Geometry check sheet. Reference: the model listing, model coordinates, mm. A direction names the side the tool comes from. Round coordinates to 2 decimals unless told otherwise and drop trailing zeros. Write each loop counter-clockwise with the first axis right and the second up, starting at its lowest first coordinate (ties: lowest second). Pieces come first, ordered by that corner, then holes. Notation, with made-up numbers: (66.25, -36) -> (100.25, -36) arc R15 ccw to (100.25, -19) -> close; hole circle Ø11 at (65, 75.25). An arc over 180 degrees is marked (long way). Use a Markdown table: item, result.
```python
from build123d import *

# Parameters (mm, degrees)
SKETCH1_R           = 12.5
BOSS_EXTRUDE1_DEPTH = 17.5
SKETCH2_R           = 2
BOSS_EXTRUDE2_DEPTH = 26
CHAMFER1_SIZE       = 10
SKETCH3_W           = 28.997372317
SKETCH3_H           = 7.197339184
CUT_EXTRUDE1_DEPTH  = 20
SKETCH4_R           = 5
CUT_EXTRUDE2_DEPTH  = 5
SKETCH5_R           = 3.5
BOSS_EXTRUDE3_DEPTH = 3.5
CUT_EXTRUDE6_START  = -1
CUT_EXTRUDE6_DEPTH  = 1


with BuildPart() as part:
    # Sketch1 → Boss-Extrude1 (new, symmetric)
    with BuildSketch(Plane(origin=(0, 0, 0), x_dir=(0, 0, -1), z_dir=(1, 0, 0))):
        Circle(SKETCH1_R)
    extrude(amount=BOSS_EXTRUDE1_DEPTH, both=True)

    # Sketch2 → Boss-Extrude2 (add, symmetric)
    with BuildSketch(Plane(origin=(0, 0, 0), x_dir=(0, 0, -1), z_dir=(1, 0, 0))):
        with Locations(Location((0, 0, 0), (0, 0, 180))):
            Circle(SKETCH2_R)
    extrude(amount=BOSS_EXTRUDE2_DEPTH, both=True)

    # Chamfer1
    chamfer1_edges = [part.edges().sort_by_distance(p)[0] for p in [
        (-17.5, 0, 12.5),
        (17.5, 0, 12.5),
    ]]
    chamfer(chamfer1_edges, length=CHAMFER1_SIZE)

    # Sketch3 → Cut-Extrude1 (cut, symmetric)
    with BuildSketch(Plane(origin=(0, 0, 0), x_dir=(0, 0, -1), z_dir=(1, 0, 0))):
        with Locations((0.644848308, -13.770631617)):
            Rectangle(SKETCH3_W, SKETCH3_H)
    extrude(amount=CUT_EXTRUDE1_DEPTH, both=True, mode=Mode.SUBTRACT)

    # Sketch4 → Cut-Extrude2 (cut)
    with BuildSketch(Plane.XZ.offset(10.171962025)):
        with Locations(Location((0, 0, 0), (0, 0, 270))):
            Circle(SKETCH4_R)
    extrude(amount=-CUT_EXTRUDE2_DEPTH, mode=Mode.SUBTRACT)

    # Sketch5 → Boss-Extrude3 (add)
    with BuildSketch(Plane.ZY.offset(26)):
        Circle(SKETCH5_R)
    boss_extrude3 = extrude(amount=BOSS_EXTRUDE3_DEPTH)

    # Sketch6 → Cut-Extrude6 (cut)
    with BuildSketch(Plane.ZY.offset(29.5).offset(CUT_EXTRUDE6_START)):
        with BuildLine():
            Line((2.803043133, -2.095936352), (-2.095936352, 2.803043133))
            ThreePointArc((-2.095936352, 2.803043133), (-2.474873734, 2.474873734), (-2.803043133, 2.095936352))
            Line((-2.803043133, 2.095936352), (2.095936352, -2.803043133))
            ThreePointArc((2.095936352, -2.803043133), (2.474873734, -2.474873734), (2.803043133, -2.095936352))
        make_face()
    cut_extrude6 = extrude(amount=CUT_EXTRUDE6_DEPTH, mode=Mode.SUBTRACT)

    # Mirror1: Boss-Extrude3, Cut-Extrude6 across plane
    add(boss_extrude3.mirror(Plane(origin=(0, 0, 0), x_dir=(0, 0, 1), z_dir=(1, 0, 0))))
    add(cut_extrude6.mirror(Plane(origin=(0, 0, 0), x_dir=(0, 0, 1), z_dir=(1, 0, 0))), mode=Mode.SUBTRACT)


solid = part.part
```
(1) Section check C-C on x = -22.5. Record the cut outline in (y, z), plus the area to 3 significant figures.
A:
| item | result |
|---|---|
| outline | circle Ø4 at (0, 0) |
| area | 12.6 mm2 |
(2) Thickness scan on line 1 (X direction, y = -8.3, z = 0); line 2 (X direction, y = -6.4, z = 0); line 3 (Y direction, x = 23, z = 1.25). Record the ranges inside material, lowest first.
A:
| item | result |
|---|---|
| line 1 | x = -11.7 to -5, 5 to 11.7 |
| line 2 | x = -13.6 to -5, 5 to 13.6 |
| line 3 | y = -1.56 to 1.56 |
(3) Release check for a two-part mould opening along Y. For faces 6 (the face through (28.993, 0.319, 0.388)), 7 (the face through (0, -5.172, 0)), 8 (the face through (-27.726, -3.105, 1.615)) record: +Y half, -Y half, draft (parallel to the pull), parting line (faces both ways), or undercut.
A:
| item | result |
|---|---|
| face 6 | undercut |
| face 7 | -Y half |
| face 8 | parting line |
(4) Gauge pin test, flat ends, axial feed: pin 1 Ø3 at (x, z) = (-8, 4.5) entering from +Y; pin 2 Ø12 at (x, z) = (17, -7) entering from +Y; pin 3 Ø6 at (x, y) = (-4.5, -2) entering from +Z; pin 4 Ø2 at (y, z) = (-7.5, -8) entering from -X. Record the tip position at first contact, or that the pin passes through.
A:
| item | result |
|---|---|
| pin 1 | stops at y = 12.11 |
| pin 2 | stops at y = 7.17 |
| pin 3 | stops at z = 12.5 |
| pin 4 | stops at x = -10.03 |
(5) Section check D-D on x = -11.5. Record the cut outline in (y, z), plus the area to 3 significant figures.
A:
| item | result |
|---|---|
| outline | circle Ø17 at (0, 0) |
| area | 227 mm2 |
(6) Access from +Z, -Z, +X, -X, +Y, -Y to the whole of each face (thin tool, end or side, straight path). Record for faces 1 (the face through (-28.993, -0.319, -0.388)), 2 (the face through (-17.5, 2, 1)), 3 (the face through (29.5, 1, 1)), 4 (the face through (28.993, -0.319, -0.388)), 5 (the face through (-4.88, -7.71, 1.08)).
A:
| item | result |
|---|---|
| face 1 | -X |
| face 2 | none |
| face 3 | +Z, -Z, +X, +Y, -Y |
| face 4 | +X |
| face 5 | -Y |
(7) Section check A-A on x = 0. Record the cut outline in (y, z).
A:
| item | result |
|---|---|
| outline | (-10.17, -7.27) arc R12.5 ccw (long way) to (-10.17, 7.27) -> (-10.17, 5) -> (-5.17, 5) -> (-5.17, -5) -> (-10.17, -5) -> close |
